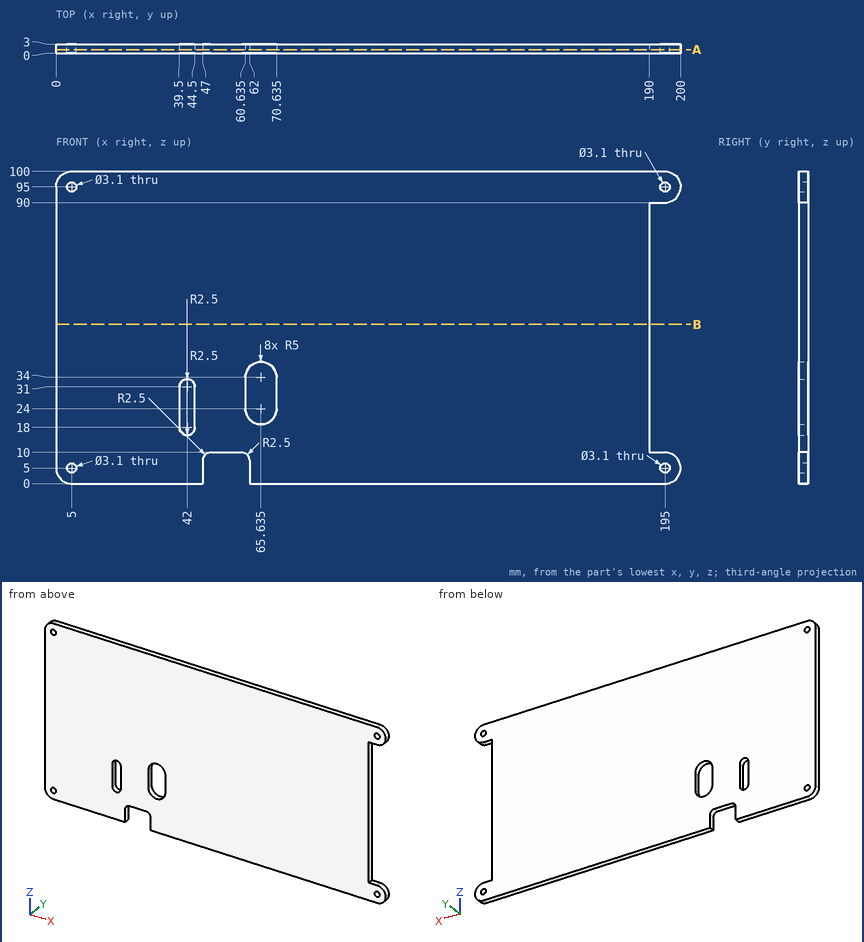
Geometry: see drawing. Coordinates: mm, zero at the bounding-box minimum. Coordinates: 2 decimals unless noted, no trailing zeros. Loops run counter-clockwise (first coordinate to the right, second up) from the corner with the lowest first, then second, coordinate; pieces in that order, holes last. Notation, with made-up numbers: M 89.25,0.25 L 112.25,0.25 A16 ccw 112.25,11.25 Z; hole C 66.5,-20.75 d5. An arc over 180 degrees is marked long. Put each result on its own line as item: value. Start each with the question number.
1) Ray query, L1, parallel to Z at x = 5, y = 1.9; L2, parallel to Z at x = 195, y = 1.3; L3, parallel to X at y = 2.05, z = 95. Return the intervals inside material, ascending. Write a range as from..to.
2) Cut plane A-A on y = 1.2. Give the number of separate pieces and of enclosed holes in the cut face, then the cut area to 3 significant figures.
3) Cut plane B-B on z = 51. Return the cut outline in (x, y), then the cut area to 3 significant figures.
4) Contact query for flat-ended pins moving along their axis: pin 1 Ø0.9 at (y, z) = (2, 22.5) entering from +X; pin 2 Ø3 at (x, z) = (195, 5) entering from -Y; pin 3 Ø1.5 at (y, z) = (1.5, 4) entering from -X. Output: stop coordinate, or through.
The answers:
1. L1: z = 0..3.45, 6.55..93.45, 96.55..100
1. L2: z = 0..3.45, 6.55..10, 90..93.45, 96.55..100
1. L3: x = 0..3.45, 6.55..193.45, 196.55..200
2. separate pieces: 1
2. enclosed holes: 6
2. area: 18,700 mm²
3. outline: M 0,0 L 190,0 L 190,3 L 0,3 Z
3. area: 570 mm²
4. pin 1: stops at x = 190
4. pin 2: passes through
4. pin 3: stops at x = 0.01
